```python
from build123d import *

# Parameters (mm, degrees)
ESQUISSE3_W                   = 53.75
ESQUISSE3_H                   = 73.333333334
BOSS_EXTRU_2_DEPTH            = 6.35
CONG_6_R                      = 20
CONG_7_R                      = 15
ESQUISSE4_R                   = 2.25
ENL_V_MAT_EXTRU_2_DEPTH       = 6.35
SYM_TRIE2_COPY_1_SKETCH_R     = 2.25
SYM_TRIE2_COPY_1_DEPTH        = 6.35
DIAM_TRE_DU_PER_AGE_4_0_4_1_D = 4


with BuildPart() as part:
    # Esquisse3 → Boss.-Extru.2 (new body)
    with BuildSketch(Plane.XY):
        Polygon((-54.672450369, 55), (54.672450369, 55), (71.992958445, 85), (107.5, 64.5), (77.5, 12.538475773), (77.5, -12.538475773), (107.5, -64.5), (71.992958445, -85), (54.672450369, -55), (-54.672450369, -55), (-71.992958445, -85), (-107.5, -64.5), (-77.5, -12.538475773), (-77.5, 12.538475773), (-107.5, 64.5), (-71.992958445, 85), align=None)
        Rectangle(ESQUISSE3_W, ESQUISSE3_H, mode=Mode.SUBTRACT)
    extrude(amount=-BOSS_EXTRU_2_DEPTH)

    # Congé6
    cong_6_edges = [part.edges().sort_by_distance(p)[0] for p in [
        (-54.672450369, 55, -3.175),
        (54.672450369, 55, -3.175),
        (77.5, 12.538475773, -3.175),
        (77.5, -12.538475773, -3.175),
        (54.672450369, -55, -3.175),
        (-54.672450369, -55, -3.175),
        (-77.5, -12.538475773, -3.175),
        (-77.5, 12.538475773, -3.175),
        (-26.875, -36.666666667, -3.175),
        (-26.875, 36.666666667, -3.175),
        (26.875, 36.666666667, -3.175),
        (26.875, -36.666666667, -3.175),
    ]]
    fillet(cong_6_edges, radius=CONG_6_R)

    # Congé7
    cong_7_edges = [part.edges().sort_by_distance(p)[0] for p in [
        (71.992958445, 85, -3.175),
        (107.5, 64.5, -3.175),
        (107.5, -64.5, -3.175),
        (71.992958445, -85, -3.175),
        (-71.992958445, -85, -3.175),
        (-107.5, -64.5, -3.175),
        (-107.5, 64.5, -3.175),
        (-71.992958445, 85, -3.175),
    ]]
    fillet(cong_7_edges, radius=CONG_7_R)

    # Esquisse4 → Enlèv. mat.-Extru.2 (cut)
    with BuildSketch(Plane.XY):
        with Locations((-56.291352203, 26.80402023)):
            Circle(ESQUISSE4_R)
        with Locations((-64.951606241, 21.80402023)):
            Circle(ESQUISSE4_R)
        with Locations((-89.201606241, 63.806252313)):
            Circle(ESQUISSE4_R)
        with Locations((-80.541352203, 68.806252313)):
            Circle(ESQUISSE4_R)
        Polygon((-53.283116293, 32.293602792), (-74.283116293, 68.666669751), (-92.209842152, 58.316669751), (-71.209842152, 21.943602792), align=None)
        with BuildLine():
            Line((-51.695036381, 4.342967697), (-54.695036381, 9.53912012))
            ThreePointArc((-54.695036381, 9.53912012), (-53.871479222, 12.612677278), (-50.797922064, 11.78912012))
            Line((-50.797922064, 11.78912012), (-47.797922064, 6.592967697))
            ThreePointArc((-47.797922064, 6.592967697), (-48.621479222, 3.519410539), (-51.695036381, 4.342967697))
        make_face()
    enl_v_mat_extru_2 = extrude(amount=-ENL_V_MAT_EXTRU_2_DEPTH, mode=Mode.SUBTRACT)

    # Symétrie1: Enlèv. mat.-Extru.2 across plane
    add(enl_v_mat_extru_2.mirror(Plane.ZX), mode=Mode.SUBTRACT)

    # Symétrie2: Enlèv. mat.-Extru.2 across plane
    add(enl_v_mat_extru_2.mirror(Plane(origin=(0, 0, 0), x_dir=(0, 0, 1), z_dir=(1, 0, 0))), mode=Mode.SUBTRACT)

    # Symétrie2 copy 1 sketch → Symétrie2 copy 1 (cut)
    with BuildSketch(Plane(origin=(0, 0, 0), x_dir=(-1, 0, 0), z_dir=(0, 0, 1))):
        with Locations((-56.291352203, 26.80402023)):
            Circle(SYM_TRIE2_COPY_1_SKETCH_R)
        with Locations((-64.951606241, 21.80402023)):
            Circle(SYM_TRIE2_COPY_1_SKETCH_R)
        with Locations((-89.201606241, 63.806252313)):
            Circle(SYM_TRIE2_COPY_1_SKETCH_R)
        with Locations((-80.541352203, 68.806252313)):
            Circle(SYM_TRIE2_COPY_1_SKETCH_R)
        Polygon((-53.283116293, 32.293602792), (-74.283116293, 68.666669751), (-92.209842152, 58.316669751), (-71.209842152, 21.943602792), align=None)
        with BuildLine():
            Line((-51.695036381, 4.342967697), (-54.695036381, 9.53912012))
            ThreePointArc((-54.695036381, 9.53912012), (-53.871479222, 12.612677278), (-50.797922064, 11.78912012))
            Line((-50.797922064, 11.78912012), (-47.797922064, 6.592967697))
            ThreePointArc((-47.797922064, 6.592967697), (-48.621479222, 3.519410539), (-51.695036381, 4.342967697))
        make_face()
    extrude(amount=-SYM_TRIE2_COPY_1_DEPTH, mode=Mode.SUBTRACT)

    # Diamètre du perçage Ø4.0 (4)1 (through all)
    with Locations(Plane.XY):
        with Locations((33, 48), (-33, 48), (-33, -48), (33, -48)):
            Hole(DIAM_TRE_DU_PER_AGE_4_0_4_1_D / 2)


solid = part.part
```
Work out the finished part from the listing and answer in its coordinate system (mm). A direction names the side the tool comes from. Round coordinates to 2 decimals unless told otherwise and drop trailing zeros.
1) Flat-ended cylindrical pins translate along their axes: P1, Ø1.5, axis at y = 39, z = -2, coming from the -X side; P2, Ø3, axis at y = 27, z = -2, coming from the -X side; P3, Ø1.9, axis at x = 2.5, z = -2.5, coming from the -Y side. Find the tip coordinate at first contact, or state that the pin passes through.
2) A cutting plane is placed at A-A on z = -3.5. Give the number of separate pieces and of enclosed holes in the cut face, and give its area (3 significant figures).
3) Which of the six approach directions +Z, -Z, +X, -X, +Y, -Y give full straight-line access (tool end or side, diameter ignored) to faces 4 (the face through (-101.54, -62.73, -3.22)), 5 (the face through (-1, 55, -3)), 6 (the face through (49.32, -9.23, -3.13))?
4) Consider probe 1 along Y at (x, z) = (33, -5); probe 2 along Y at (x, z) = (-80, -3.5); probe 3 along X at (y, z) = (-27, -0.25). Determine where each line is inside the solid, lowest interval first.
5) Determine the mould class of faces 1 (the face through (66.61, 23.325, -3.131)), 2 (the face through (78.2, 12.43, -3.22)), 3 (the face through (-90.228, -34.585, -3.131)) for opening direction X: pulls with the +X half, pulls with the -X half, needs draft (parallel to the pull), parting line crosses it, or undercut.
Entries:
1. P1: stops at x = -93.21
1. P2: stops at x = -86.72
1. P3: stops at y = -55
2. separate pieces: 1
2. enclosed holes: 29
2. area: 15,000 mm2
3. face 4: +Z, -Z, -X
3. face 5: +Z, -Z, +Y
3. face 6: +Z, -Z
4. probe 1: y = -55 to -50, -46 to 46, 50 to 55
4. probe 2: y = -79.3 to -70.99, -66.62 to -65.37, -37.17 to -16.86, 16.86 to 37.17, 65.37 to 66.62, 70.99 to 79.3
4. probe 3: x = -85.85 to -74.13, -62.45 to -58.53, -54.05 to -24, 24 to 54.05, 58.53 to 62.45, 74.13 to 85.85
5. face 1: undercut
5. face 2: pulls with the +X half
5. face 3: pulls with the -X half
